Work out the finished part from the listing and answer in its coordinate system (mm). Face numbers are marked on the shaded views. Coordinates: 2 decimals unless noted, no trailing zeros. Order: outer loops, then holes, each group sorted by start corner. A loop starts at its lowest first (then second) coordinate and runs counter-clockwise, first axis right, second up. Notation, with made-up numbers: M -35.5,-36 L -15.5,-36 A28 ccw -15.5,-12 Z; hole C 17,-0.5 d1. An arc over 180 degrees is marked long. Write item = value, one per line. Start each with the question number.
Q1. Determine the mould class of the marked faces 1, 2, 3 and 4 for opening direction X: released by +X, released by -X, zero draft, split by the parting line, or undercut.
Q2. Find section A-A on x = 12.5. Give the vertices of the cut face in (y, z), and give its area (3 significant figures).
Q3. Each of these flat-tipped pins is pushed along its axis until it touches: P1, Ø3, axis at x = -23, z = -9, coming from the -Y side; P2, Ø8, axis at y = 7.5, z = -13, coming from the +X side; P3, Ø1.2, axis at x = -23, z = -17, coming from the +Y side. Where does it stop, or does it pass through?
Q4. Find section D-D on y = 18. Give the vertices of the cut face in (x, z).
Q5. Straight lines are drawn through the part: line 1 along X through (y, z) = (1.5, -20); line 2 along Y through (x, z) = (-12.5, 1.15); line 3 along Z through (x, y) = (2.5, 12). For each, find the intervals that lie inside material, in ascending order.
Q6. Find section B-B on z = -20.75. Give the vertices of the cut face in (x, y).
Q7. Find section C-C on y = -17.5. Give the vertices of the cut face in (x, z).
```python
from build123d import *

# Parameters (mm, degrees)
SKETCH009_W     = 54
SKETCH009_H     = 54
PAD002_DEPTH    = 2
SKETCH008_R     = 6.25
SKETCH008_W     = 33
SKETCH008_H     = 18.3
POCKET006_DEPTH = 2
SKETCH013_R     = 1.5
PAD004_DEPTH    = 1.5
SKETCH014_W     = 4
SKETCH014_H     = 23
PAD005_DEPTH    = 25
CHAMFER001_SIZE = 1


with BuildPart() as part:
    # Sketch009 → Pad002 (new body)
    with BuildSketch(Plane.XY):
        Rectangle(SKETCH009_W, SKETCH009_H)
    extrude(amount=PAD002_DEPTH)

    # Sketch008 (on Face6 of Pad002) → Pocket006 (cut)
    with BuildSketch(Plane.XY.offset(2)):
        with Locations((-12.5, 18)):
            Circle(SKETCH008_R)
        with Locations((12.5, 18)):
            Circle(SKETCH008_R)
        with Locations((0, -10.15)):
            Rectangle(SKETCH008_W, SKETCH008_H)
    extrude(amount=-POCKET006_DEPTH, mode=Mode.SUBTRACT)

    # Sketch013 (on Face4 of Pocket006) → Pad004 (join)
    with BuildSketch(Plane(origin=(0, 0, 0), x_dir=(1, 0, 0), z_dir=(0, 0, -1))):
        with Locations((-15.24, 21.71)):
            Circle(SKETCH013_R)
        with Locations((15.24, 21.71)):
            Circle(SKETCH013_R)
        with Locations((15.24, -6.23)):
            Circle(SKETCH013_R)
        with Locations((-15.24, -6.23)):
            Circle(SKETCH013_R)
    extrude(amount=PAD004_DEPTH)

    # Sketch014 (on Face4 of Pad004) → Pad005 (join)
    with BuildSketch(Plane(origin=(0, 0, 0), x_dir=(1, 0, 0), z_dir=(0, 0, -1))):
        with Locations((-22.86, -7.68)):
            Rectangle(SKETCH014_W, SKETCH014_H)
        with Locations((22.86, -7.68)):
            Rectangle(SKETCH014_W, SKETCH014_H)
    extrude(amount=PAD005_DEPTH)

    # Chamfer001
    chamfer001_edges = [part.edges().sort_by_distance(p)[0] for p in [
        (0, -19.3, 2),
        (-16.5, -10.15, 2),
        (0, -1, 2),
        (16.5, -10.15, 2),
    ]]
    chamfer(chamfer001_edges, length=CHAMFER001_SIZE)


solid = part.part
```
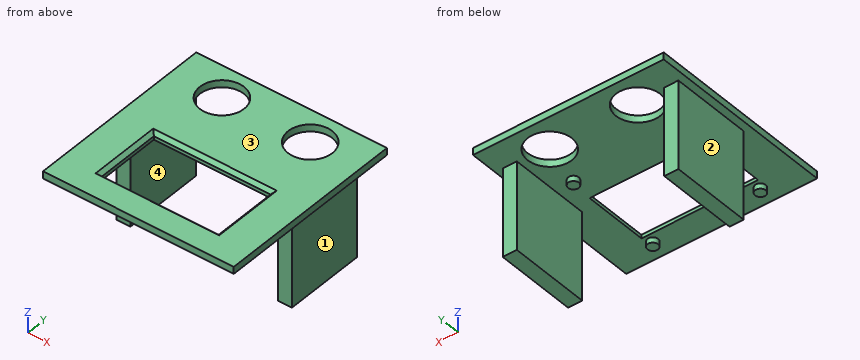
Findings below:
q1.face_1 = released by +X
q1.face_2 = released by -X
q1.face_3 = zero draft
q1.face_4 = undercut
q2.outline = M -27,0 L -19.3,0 L -19.3,1 L -20.3,2 L -27,2 Z; M -1,0 L 11.75,0 L 11.75,2 L 0,2 L -1,1 Z; M 24.25,0 L 27,0 L 27,2 L 24.25,2 Z
q2.area = 45.4 mm^2
q3.P1 = -3.82
q3.P2 = 24.86
q3.P3 = 19.18
q4.outline = M -27,0 L -24.86,0 L -24.86,-25 L -20.86,-25 L -20.86,0 L -18.75,0 L -18.75,2 L -27,2 Z; M -6.25,0 L 6.25,0 L 6.25,2 L -6.25,2 Z; M 18.75,0 L 20.86,0 L 20.86,-25 L 24.86,-25 L 24.86,0 L 27,0 L 27,2 L 18.75,2 Z
q5.line_1 = -24.86 to -20.86, 20.86 to 24.86
q5.line_2 = -27 to -19.45, -0.85 to 11.75, 24.25 to 27
q5.line_3 = 0 to 2
q6.outline = M -24.86,-3.82 L -20.86,-3.82 L -20.86,19.18 L -24.86,19.18 Z; M 20.86,-3.82 L 24.86,-3.82 L 24.86,19.18 L 20.86,19.18 Z
q7.outline = M -27,0 L -16.5,0 L -16.5,1 L -17.5,2 L -27,2 Z; M 16.5,0 L 27,0 L 27,2 L 17.5,2 L 16.5,1 Z
